Autodesk Inventor part; units mm, degrees
ref_plane "YZ Plane" through (0, 0, 0) normal (1, 0, 0) x (0, 1, 0)
ref_plane "XZ Plane" through (0, 0, 0) normal (0, 1, 0) x (-1, 0, 0)
ref_plane "XY Plane" through (0, 0, 0) normal (0, 0, 1) x (1, 0, 0)
ref_plane "РабПлоскость2" through (0, 0, -70) normal (0, 0, -1) x (-1, 0, 0)
sketch "Эскиз4" plane through (0, 0, 0) normal (1, 0, 0) x (0, 1, 0)
  line L0 (-2, -70) -> (2, -70)
  line L1 (-50, -180) -> (-120, -180)
  arc A0 (-50, -180) -> (0, -130) centre (-50, -130) ccw
  line L2 (0, -130) -> (0, -70)
  line L3 (2, -70) -> (-250, -70) construction
  dimension "d9" = 60
  dimension "d11" = 50
  dimension "d13" = 70
sketch "Эскиз5" plane through (0, 0, -70) normal (0, 0, -1) x (-1, 0, 0)
  circle A0 centre (0, 0) radius 1
  circle A1 centre (0, 0) radius 2
sweep "Сдвиг2" add profiles "Эскиз5" path "Эскиз4" path curves L2 A0 L1
properties part number "тефлон"
Geometry check sheet. Reference: the model listing, model coordinates, mm. Coordinates: 2 decimals unless noted, no trailing zeros. Order: outer loops, then holes, each group sorted by start corner. A loop starts at its lowest first (then second) coordinate and runs counter-clockwise, first axis right, second up.
Item 1: Depth check by flat-ended pin: pin 1 (1.5 mm diameter, centred on x = 1, z = -97, fed in from +Y). Enter the tip coordinate at first touch or a pass-through.
Item 2: Section check C-C (y = -90.5). Enter the section's corners in (x, z).
Item 3: Scan lines: line 1 along Y through (x, z) = (0, -85); line 2 along Z through (x, y) = (0, -66.5). Record each from-to range of solid material in increasing order.
Item 4: Mould release check, pull along Y, two halves, no side actions. Record for faces 1 (the cylindrical face through (-0.923, -84.51, -181.774)), 2 (the flat face through (-1, -120, -181)), 3 (the cylindrical face through (0, 2, -100)): released by +Y, released by -Y, zero draft, split by the parting line, or undercut.
Item 5: Section check A-A (x = 0). Enter the section's corners in (y, z).
Item 6: Section check B-B (z = -104). Enter the section's corners in (x, y).
Check sheet entries:
1. pin 1: stops at y = 1.98
2. outline: circle Ø4 at (0, -180); hole circle Ø2 at (0, -180)
3. line 1: y = -2 to -1, 1 to 2
3. line 2: z = -182 to -181, -179 to -178
4. face 1: zero draft
4. face 2: released by -Y
4. face 3: split by the parting line
5. outline: (-120, -182) - (-50, -182) arc R52 ccw to (2, -130) - (2, -70) - (1, -70) - (1, -130) arc R51 cw to (-50, -181) - (-120, -181) - close; (-120, -179) - (-50, -179) arc R49 ccw to (-1, -130) - (-1, -70) - (-2, -70) - (-2, -130) arc R48 cw to (-50, -178) - (-120, -178) - close
6. outline: circle Ø4 at (0, 0); hole circle Ø2 at (0, 0)
